from build123d import *

# Parameters (mm, degrees)
BOSS_EXTRUDE1_DEPTH = 152.4


with BuildPart() as part:
    # Sketch1 → Boss-Extrude1 (new body, symmetric)
    with BuildSketch(Plane(origin=(0, 0, 0), x_dir=(1, 0, 0), z_dir=(0, 1, 0))):
        with BuildLine():
            Line((-50.8, -76.2), (50.8, -76.2))
            ThreePointArc((50.8, -76.2), (68.760512242, -68.760512242), (76.2, -50.8))
            Line((76.2, -50.8), (76.2, 50.8))
            ThreePointArc((76.2, 50.8), (68.760512242, 68.760512242), (50.8, 76.2))
            Line((50.8, 76.2), (-50.8, 76.2))
            ThreePointArc((-50.8, 76.2), (-68.760512242, 68.760512242), (-76.2, 50.8))
            Line((-76.2, 50.8), (-76.2, -50.8))
            ThreePointArc((-76.2, -50.8), (-68.760512242, -68.760512242), (-50.8, -76.2))
        make_face()
        with BuildLine():
            Line((-50.8, -63.5), (50.8, -63.5))
            ThreePointArc((50.8, -63.5), (59.780256121, -59.780256121), (63.5, -50.8))
            Line((63.5, -50.8), (63.5, 50.8))
            ThreePointArc((63.5, 50.8), (59.780256121, 59.780256121), (50.8, 63.5))
            Line((50.8, 63.5), (-50.8, 63.5))
            ThreePointArc((-50.8, 63.5), (-59.780256121, 59.780256121), (-63.5, 50.8))
            Line((-63.5, 50.8), (-63.5, -50.8))
            ThreePointArc((-63.5, -50.8), (-59.780256121, -59.780256121), (-50.8, -63.5))
        make_face(mode=Mode.SUBTRACT)
    extrude(amount=BOSS_EXTRUDE1_DEPTH, both=True)


solid = part.part
Could you check a few things on this model? Use its own coordinates, in mm. A direction names the side the tool comes from. Give positions to 0.01 mm unless a question says otherwise; leave off trailing zeros. Order: outer loops, then holes, each group sorted by start corner. A loop starts at its lowest first (then second) coordinate and runs counter-clockwise, first axis right, second up. Notation, with made-up numbers: (43, 83.5) -> (74, 83.5) arc R30 ccw to (74, 111.5) -> close; hole circle Ø1 at (46, 49). An arc over 180 degrees is marked (long way). Answer in a Markdown table with one row per item. Add a question column.
Item 1: Imagine slicing it at A-A (z = -13.5). List the corners of the cut face in (x, y) for me, and give its area (3 significant figures).
Item 2: For faces 4 (the cylindrical face through (68.96, 2.13, -68.56)), 5 (the cylindrical face through (59.68, 2.13, 59.88)), which set-ups out of +Z, -Z, +X, -X, +Y, -Y let a thin tool reach every point of the face, with its end or its side?
Item 3: We'd pull the mould along Z, two halves only. Please class faces 1 (the flat face through (1, 2, -63.5)), 2 (the flat face through (-1, -152.4, 67)), 3 (the cylindrical face through (68.56, 2.13, 68.96)): pulls with the +Z half, pulls with the -Z half, needs draft (parallel to the pull), parting line crosses it, or undercut.
Item 4: I'm going to push a flat-ended pin straight in: P1, Ø6, axis at x = 57.5, y = 47, coming from the +Z side. Where does the tip first touch, or does it pass through?
Item 5: Imagine slicing it at B-B (x = -39). List the corners of the cut face in (y, z) for me.
Item 6: Please list where these lines run through material, in increasing order: probe 1 along X at (y, z) = (57, -5); probe 2 along X at (y, z) = (116, -60) (3 decimals).
Item 7: Imagine slicing it at C-C (y = 27.5). List the corners of the cut face in (x, z) for me, and give its area (3 significant figures).
Result:
| question | item | result |
|---|---|---|
| 1 | outline | (-76.2, -152.4) -> (-63.5, -152.4) -> (-63.5, 152.4) -> (-76.2, 152.4) -> close; (63.5, -152.4) -> (76.2, -152.4) -> (76.2, 152.4) -> (63.5, 152.4) -> close |
| 1 | area | 7,740 mm2 |
| 2 | face 4 | -Z, +X, +Y, -Y |
| 2 | face 5 | +Y, -Y |
| 3 | face 1 | undercut |
| 3 | face 2 | needs draft |
| 3 | face 3 | pulls with the +Z half |
| 4 | P1 | z = 75.93 |
| 5 | outline | (-152.4, -76.2) -> (152.4, -76.2) -> (152.4, -63.5) -> (-152.4, -63.5) -> close; (-152.4, 63.5) -> (152.4, 63.5) -> (152.4, 76.2) -> (-152.4, 76.2) -> close |
| 6 | probe 1 | -76.2 to -63.5, 63.5 to 76.2 |
| 6 | probe 2 | -74.475 to -59.555, 59.555 to 74.475 |
| 7 | outline | (-76.2, -50.8) arc R25.4 ccw to (-50.8, -76.2) -> (50.8, -76.2) arc R25.4 ccw to (76.2, -50.8) -> (76.2, 50.8) arc R25.4 ccw to (50.8, 76.2) -> (-50.8, 76.2) arc R25.4 ccw to (-76.2, 50.8) -> close; hole (-63.5, -50.8) arc R12.7 ccw to (-50.8, -63.5) -> (50.8, -63.5) arc R12.7 ccw to (63.5, -50.8) -> (63.5, 50.8) arc R12.7 ccw to (50.8, 63.5) -> (-50.8, 63.5) arc R12.7 ccw to (-63.5, 50.8) -> close |
| 7 | area | 6,680 mm2 |
